Could you check a few things on this model? Use its own coordinates, in mm. A direction names the side the tool comes from. Give positions to 0.01 mm unless a question says otherwise; leave off trailing zeros. Loops run counter-clockwise (first coordinate to the right, second up) from the corner with the lowest first, then second, coordinate; pieces in that order, holes last. Notation, with made-up numbers: (55, 30.25) - (95, 30.25) arc R21 ccw to (95, 52.25) - close; hole circle Ø9 at (87, -33). An arc over 180 degrees is marked (long way). Write each question's results on one line, items separated by ' | '. Start each with the question number.
```python
from build123d import *

# Parameters (mm, degrees)
SKETCH1_W            = 50.8
SKETCH1_H            = 50.8
BOSS_EXTRUDE1_DEPTH  = 1.5875
SKETCH3_R            = 1.2065
BOSS_EXTRUDE2_DEPTH  = 8.89
SKETCH4_R            = 2.54
CUT_EXTRUDE1_DEPTH   = 43.790708396
BOSS_EXTRUDE3_START  = 12.065
SKETCH5_R            = 1.2065
BOSS_EXTRUDE3_DEPTH  = 12.065
M2_CLEARANCE_HOLE1_D = 2.6
CUT_EXTRUDE2_REACH   = 47.375
SKETCH8_W            = 5.08
SKETCH8_H            = 21.59


with BuildPart() as part:
    # Sketch1 → Boss-Extrude1 (new, symmetric)
    with BuildSketch(Plane(origin=(0, 0, 0), x_dir=(1, 0, 0), z_dir=(0, 1, 0))):
        Rectangle(SKETCH1_W, SKETCH1_H)
    extrude(amount=BOSS_EXTRUDE1_DEPTH, both=True)

    # Sketch3 → Boss-Extrude2 (add)
    with BuildSketch(Plane(origin=(25.4, 0, 0), x_dir=(0, 0, -1), z_dir=(1, 0, 0))):
        with Locations(Location((0, 0, 0), (0, 0, 180))):
            Circle(SKETCH3_R)
    extrude(amount=BOSS_EXTRUDE2_DEPTH)

    # Sketch4 → Cut-Extrude1 (cut, through all)
    with BuildSketch(Plane(origin=(0, 1.5875, 0), x_dir=(1, 0, 0), z_dir=(0, 1, 0))):
        with Locations(Location((-16.51, 16.51, 0), (0, 0, 270))):
            Circle(SKETCH4_R)
        with Locations(Location((16.51, 16.51, 0), (0, 0, 270))):
            Circle(SKETCH4_R)
        with Locations(Location((16.51, -16.51, 0), (0, 0, 270))):
            Circle(SKETCH4_R)
        with Locations(Location((-16.51, -16.51, 0), (0, 0, 270))):
            Circle(SKETCH4_R)
    extrude(amount=-CUT_EXTRUDE1_DEPTH, mode=Mode.SUBTRACT)

    # Sketch5 → Boss-Extrude3 (add)
    with BuildSketch(Plane.ZY.offset(25.4).offset(BOSS_EXTRUDE3_START)):
        Circle(SKETCH5_R)
    extrude(amount=-BOSS_EXTRUDE3_DEPTH)

    # M2 Clearance Hole1 (through all)
    with Locations(Plane(origin=(0, 1.5875, 0), x_dir=(1, 0, 0), z_dir=(0, 1, 0))):
        with Locations((-16.51, -7.62), (-16.51, 7.62), (5.08, -7.62), (5.08, 7.62), (22.86, 7.62), (22.86, -7.62)):
            Hole(M2_CLEARANCE_HOLE1_D / 2)

    # Sketch8 → Cut-Extrude2 (cut, up to next)
    with BuildSketch(Plane(origin=(0, 1.5875, 0), x_dir=(1, 0, 0), z_dir=(0, 1, 0)), mode=Mode.PRIVATE) as cut_extrude2_sk1:
        with Locations((9.906, 0.232205857)):
            Rectangle(SKETCH8_W, SKETCH8_H)
    cut_extrude2_tool1 = extrude(cut_extrude2_sk1.sketch, amount=-CUT_EXTRUDE2_REACH, mode=Mode.PRIVATE) & part.part
    add(cut_extrude2_tool1.solids().sort_by_distance((9.906, 1.5875, -0.232206))[0], mode=Mode.SUBTRACT)


solid = part.part
```
Q1. I want a section at A-A, the plane y = 0. State how many separate pieces and enclosed holes the cut face has, then the cut area to 3 significant figures.
Q2. I want a section at D-D, the plane z = -7.62. List the corners of the cut face in (x, y) for me.
Q3. I want a section at C-C, the plane z = 4.5. List the corners of the cut face in (x, y) for me.
Q4. I want a section at B-B, the plane x = -16.51. List the corners of the cut face in (y, z) for me.
Q5. I'm going to push flat-ended pins straight in: pin 1 Ø1.6 at (y, z) = (-0.5, 11.5) entering from +X; pin 2 Ø3 at (x, z) = (-16.51, -16.51) entering from +Y; pin 3 Ø1 at (y, z) = (0, -12.5) entering from -X. Where does each tip first touch, or does it pass through?
Q6. Which directions (+Z, -Z, +X, -X, +Y, -Y) give clear straight access to the entire face, cutting with the end or side of a thin tool? Please do faces 1 (the face through (0, 0, -25.4)), 2 (the face through (-31.52, -0.73, -0.96)), 3 (the face through (10, 0, -11.027)).
Q7. If we mould it in two halves opening along X, with no side actions, what happens to faces 4 (the face through (24.16, -0.02, 7.56)), 5 (the face through (29.78, 0.73, -0.96)), 6 (the face through (-25.4, -1.4, 0.4))? For each: +X half, -X half, draft (parallel to the pull), parting line (faces both ways), or undercut.
Q8. I need wall thicknesses on L1, parallel to Z at x = 5, y = -0.8; L2, parallel to X at y = -0.75, z = -16.51; L3, parallel to Z at x = 11.5, y = 0.45. Which ranges of each line are inside material? Lowest first, please. Write a range as from..to.
Conclusion:
1) separate pieces: 1 | enclosed holes: 11 | area: 2,410 mm^2
2) outline: (-25.4, -1.59) - (-17.81, -1.59) - (-17.81, 1.59) - (-25.4, 1.59) - close; (-15.21, -1.59) - (3.78, -1.59) - (3.78, 1.59) - (-15.21, 1.59) - close; (6.38, -1.59) - (7.37, -1.59) - (7.37, 1.59) - (6.38, 1.59) - close; (12.45, -1.59) - (21.56, -1.59) - (21.56, 1.59) - (12.45, 1.59) - close; (24.16, -1.59) - (25.4, -1.59) - (25.4, 1.59) - (24.16, 1.59) - close
3) outline: (-25.4, -1.59) - (7.37, -1.59) - (7.37, 1.59) - (-25.4, 1.59) - close; (12.45, -1.59) - (25.4, -1.59) - (25.4, 1.59) - (12.45, 1.59) - close
4) outline: (-1.59, -25.4) - (1.59, -25.4) - (1.59, -19.05) - (-1.59, -19.05) - close; (-1.59, -13.97) - (1.59, -13.97) - (1.59, -8.92) - (-1.59, -8.92) - close; (-1.59, -6.32) - (1.59, -6.32) - (1.59, 6.32) - (-1.59, 6.32) - close; (-1.59, 8.92) - (1.59, 8.92) - (1.59, 13.97) - (-1.59, 13.97) - close; (-1.59, 19.05) - (1.59, 19.05) - (1.59, 25.4) - (-1.59, 25.4) - close
5) pin 1: x = 25.4 | pin 2: through | pin 3: x = -25.4
6) face 1: -Z, +X, -X, +Y, -Y | face 2: -X | face 3: +Y, -Y
7) face 4: undercut | face 5: draft | face 6: -X half
8) L1: -25.4..-8.92, -6.32..6.32, 8.92..25.4 | L2: -25.4..-19.05, -13.97..13.97, 19.05..25.4 | L3: -25.4..-11.03, 10.56..25.4
